from build123d import *

# Parameters (mm, degrees)
SKETCH_1_W      = 90
SKETCH_1_H      = 15
SKETCH_1_R      = 1.5
SKETCH_1_R_2    = 2
EXTRUDE_1_DEPTH = 3


with BuildPart() as part:
    # 草图1 → 凸台-拉伸1 (new body)
    with BuildSketch(Plane.XY):
        Rectangle(SKETCH_1_W, SKETCH_1_H)
        with Locations((-13.5, 0)):
            Circle(SKETCH_1_R, mode=Mode.SUBTRACT)
        with Locations(Location((13.5, 0, 0), (0, 0, 180))):
            Circle(SKETCH_1_R, mode=Mode.SUBTRACT)
        with Locations((-39, 0)):
            Circle(SKETCH_1_R_2, mode=Mode.SUBTRACT)
        with Locations(Location((39, 0, 0), (0, 0, 180))):
            Circle(SKETCH_1_R_2, mode=Mode.SUBTRACT)
    extrude(amount=EXTRUDE_1_DEPTH)


solid = part.part
Source: CAD feature listing. Evaluate the final solid. Frame: model axes, mm. Round coordinates to 2 decimals unless told otherwise and drop trailing zeros. Loops run counter-clockwise (first coordinate to the right, second up) from the corner with the lowest first, then second, coordinate; pieces in that order, holes last.
Q1. Section B-B, the plane x = -13.5. Return loops of the section in (y, z), plus the area to 3 significant figures.
Q2. Section A-A, the plane y = 0. Return loops of the section in (x, z), plus the area to 3 significant figures.
Q3. Mould query, pull axis Y, two halves, no side actions, for faces 1 (the face through (15, 0, 1)), 2 (the face through (-1, 7.5, 1)), 3 (the face through (-45, 0, 1)). Classes: pulls with the +Y half, pulls with the -Y half, needs draft (parallel to the pull), parting line crosses it, or undercut.
Q4. Section C-C, the plane z = 1.2. Return loops of the section in (x, y), plus the area to 3 significant figures.
Q5. First-contact query: P1, Ø3, axis at x = 39, y = 0, coming from the +Z side. Flat tip, straight axial feed; report the tip coordinate or a pass-through.
Q6. Ray query, line 1 (X direction, y = -0.75, z = 0.25); line 2 (Y direction, x = 13.5, z = 1); line 3 (X direction, y = -0.25, z = 0.4). Return the intervals inside material, ascending.
Q7. Section D-D, the plane x = -39. Return loops of the section in (y, z), plus the area to 3 significant figures.
Solutions:
1. outline: (-7.5, 0) - (-1.5, 0) - (-1.5, 3) - (-7.5, 3) - close; (1.5, 0) - (7.5, 0) - (7.5, 3) - (1.5, 3) - close
1. area: 36.0 mm2
2. outline: (-45, 0) - (-41, 0) - (-41, 3) - (-45, 3) - close; (-37, 0) - (-15, 0) - (-15, 3) - (-37, 3) - close; (-12, 0) - (12, 0) - (12, 3) - (-12, 3) - close; (15, 0) - (37, 0) - (37, 3) - (15, 3) - close; (41, 0) - (45, 0) - (45, 3) - (41, 3) - close
2. area: 228 mm2
3. face 1: undercut
3. face 2: pulls with the +Y half
3. face 3: needs draft
4. outline: (-45, -7.5) - (45, -7.5) - (45, 7.5) - (-45, 7.5) - close; hole circle Ø4 at (-39, 0); hole circle Ø3 at (-13.5, 0); hole circle Ø3 at (13.5, 0); hole circle Ø4 at (39, 0)
4. area: 1,310 mm2
5. P1: passes through
6. line 1: x = -45 to -40.85, -37.15 to -14.8, -12.2 to 12.2, 14.8 to 37.15, 40.85 to 45
6. line 2: y = -7.5 to -1.5, 1.5 to 7.5
6. line 3: x = -45 to -40.98, -37.02 to -14.98, -12.02 to 12.02, 14.98 to 37.02, 40.98 to 45
7. outline: (-7.5, 0) - (-2, 0) - (-2, 3) - (-7.5, 3) - close; (2, 0) - (7.5, 0) - (7.5, 3) - (2, 3) - close
7. area: 33.0 mm2
